from build123d import *

# Parameters (mm, degrees)
SKETCH1_W           = 50
SKETCH1_H           = 50
BOSS_EXTRUDE1_DEPTH = 10
SKETCH2_W           = 40
SKETCH2_H           = 40
CUT_EXTRUDE1_DEPTH  = 7
FILLET1_R           = 3
SKETCH3_R           = 5
SKETCH3_R_2         = 3
BOSS_EXTRUDE2_DEPTH = 5


with BuildPart() as part:
    # Sketch1 → Boss-Extrude1 (new body)
    with BuildSketch(Plane(origin=(0, 0, 0), x_dir=(1, 0, 0), z_dir=(0, 1, 0))):
        with Locations((25, 25)):
            Rectangle(SKETCH1_W, SKETCH1_H)
    extrude(amount=BOSS_EXTRUDE1_DEPTH)

    # Sketch2 → Cut-Extrude1 (cut)
    with BuildSketch(Plane(origin=(0, 10, 0), x_dir=(1, 0, 0), z_dir=(0, 1, 0))):
        with Locations((25, 25)):
            Rectangle(SKETCH2_W, SKETCH2_H)
    extrude(amount=-CUT_EXTRUDE1_DEPTH, mode=Mode.SUBTRACT)

    # Fillet1
    fillet1_edges = [part.edges().sort_by_distance(p)[0] for p in [
        (5, 3, -25),
        (25, 3, -45),
        (45, 3, -25),
        (25, 3, -5),
    ]]
    fillet(fillet1_edges, radius=FILLET1_R)

    # Sketch3 → Boss-Extrude2 (add)
    with BuildSketch(Plane(origin=(0, 3, 0), x_dir=(1, 0, 0), z_dir=(0, 1, 0))):
        with Locations(Location((19, 35, 0), (0, 0, 270))):
            Circle(SKETCH3_R)
        with Locations(Location((32, 25, 0), (0, 0, 270))):
            Circle(SKETCH3_R)
        with Locations(Location((15, 25, 0), (0, 0, 270))):
            Circle(SKETCH3_R)
        with Locations(Location((32, 12, 0), (0, 0, 270))):
            Circle(SKETCH3_R_2)
    extrude(amount=BOSS_EXTRUDE2_DEPTH)


solid = part.part
CAD build for the part. Positions are in the model's coordinates, mm. A direction names the side the tool comes from. Give positions to 0.01 mm unless a question says otherwise; leave off trailing zeros. Order: outer loops, then holes, each group sorted by start corner. A loop starts at its lowest first (then second) coordinate and runs counter-clockwise, first axis right, second up. Notation, with made-up numbers: (20, 15) - (43, 15) arc R31 cw to (43, 51) - close; hole circle Ø5 at (82, 49). An arc over 180 degrees is marked (long way). Write each question's results on one line, items separated by ' | '.
1. 3-axis set-ups, long thin cutter, end or side, ignore diameter. For faces 1 (the face through (5, 8, -25)), 2 (the face through (25, 5, 0)): which of +Z, -Z, +X, -X, +Y, -Y reach the whole face in a straight line?
Calculated:
face 1: +Y | face 2: +Z, +X, -X, +Y, -Y
2. Saw through at B-B on x = 39. List the corners of the cut face in (y, z), and give its area (3 significant figures).
Calculated:
outline: (0, -50) - (10, -50) - (10, -45) - (6, -45) arc R3 cw to (3, -42) - (3, -8) arc R3 cw to (6, -5) - (10, -5) - (10, 0) - (0, 0) - close | area: 224 mm2
3. Saw through at D-D on x = 15. List the corners of the cut face in (y, z).
Calculated:
outline: (0, -50) - (10, -50) - (10, -45) - (6, -45) arc R3 cw to (3, -42) - (3, -38) - (8, -38) - (8, -32) - (3, -32) - (3, -30) - (8, -30) - (8, -20) - (3, -20) - (3, -8) arc R3 cw to (6, -5) - (10, -5) - (10, 0) - (0, 0) - close
4. Saw through at C-C on z = -12. List the corners of the cut face in (x, y).
Calculated:
outline: (0, 0) - (50, 0) - (50, 10) - (45, 10) - (45, 6) arc R3 cw to (42, 3) - (35, 3) - (35, 8) - (29, 8) - (29, 3) - (8, 3) arc R3 cw to (5, 6) - (5, 10) - (0, 10) - close
5. Saw through at A-A on y = 6.75. List the corners of the cut face in (x, z).
Calculated:
outline: (0, -50) - (50, -50) - (50, 0) - (0, 0) - close; circle Ø10 at (15, -25); circle Ø10 at (19, -35); circle Ø10 at (32, -25); circle Ø6 at (32, -12); hole (5, -45) - (45, -45) - (45, -5) - (5, -5) - close
6. Probe L1, parallel to X at y = 7.75, z = -25; L2, parallel to Z at x = 24.5, y = 8.25; L3, parallel to X at y = 8.25, z = -44. List the from-to ranges inside material, lowest first. Write a range as from..to.
Calculated:
L1: x = 0..5, 10..20, 27..37, 45..50 | L2: z = -50..-45, -5..0 | L3: x = 0..5, 45..50
7. Pin check, flat tips, straight feed: pin 1 (5 mm diameter, centred on x = 16.5, z = -25.5, fed in from +Y); pin 2 (4 mm diameter, centred on y = 2, z = -6.5, fed in from -X); pin 3 (5 mm diameter, centred on x = 37.5, z = -8, fed in from +Y); pin 4 (3 mm diameter, centred on x = 35.5, z = -39, fed in from +Y). Stop position of each tip, or through.
Calculated:
pin 1: stops at y = 8 | pin 2: stops at x = 0 | pin 3: stops at y = 4.34 | pin 4: stops at y = 3
8. Pull direction Z, two halves, no side cores. Call faces 3 (the face through (32, 5, -30)), 4 (the face through (25, 8, -5)), 5 (the face through (47, 10, -25)), 6 (the face through (25, 5, -50)): released by +Z, released by -Z, zero draft, split by the parting line, or undercut.
Calculated:
face 3: undercut | face 4: undercut | face 5: zero draft | face 6: released by -Z
